Autodesk Inventor part; units mm, degrees
ref_plane "YZ Plane" through (0, 0, 0) normal (1, 0, 0) x (0, 1, 0)
ref_plane "XZ Plane" through (0, 0, 0) normal (0, 1, 0) x (-1, 0, 0)
ref_plane "XY Plane" through (0, 0, 0) normal (0, 0, 1) x (1, 0, 0)
sketch "Sketch1" plane through (0, 0, 0) normal (1, 0, 0) x (0, 1, 0)
  line L0 (0, 0) -> (0, -24)
  line L1 (0, -24) -> (20, -24)
  line L2 (20, -24) -> (20, -20.7846)
  line L3 (20, -20.7846) -> (8, 0)
  line L4 (8, 0) -> (0, 0)
  dimension "d0" = 120
  dimension "d1" = 24
  dimension "d2" = 8
  dimension "d3" = 20
extrude "Extrusion1" add sketch "Sketch1" along normal blind 32
sketch "Sketch3" plane through (0, 8, 0) normal (0, 0.866, 0.5) x (1, 0, 0)
  circle A0 centre (8, 20) radius 3.6
  circle A1 centre (24, 20) radius 3.6
  circle A2 centre (24, 4) radius 3.6
  circle A3 centre (8, 4) radius 3.6
  line L0 (0, 0) -> (32, 0)
  line L1 (32, 24) -> (32, 0)
  line L2 (0, 24) -> (32, 24)
  circle A4 centre (16, 12) radius 3.7
  point P0 (0, -4)
  dimension "d17" = 7.2
  dimension "d18" = 7.2
  dimension "d19" = 7.2
  dimension "d20" = 7.2
  dimension "d21" = 16
  dimension "d22" = 16
  dimension "d23" = 16
  dimension "d25" = 8
  dimension "d26" = 4
  dimension "d29" = 7.4
  dimension "d30" = 8
  dimension "d31" = 8
extrude "Extrusion2" cut sketch "Sketch3" against normal through all contours A0 | A1 | A2 | A3
extrude "Extrusion3" cut sketch "Sketch3" against normal blind 6 contours A4
sketch "Sketch4" plane through (0, 8, 0) normal (0, 0.866, 0.5) x (1, 0, 0)
  circle A0 centre (24, 20) radius 2
  circle A1 centre (8, 20) radius 2
  circle A2 centre (24, 4) radius 2
  circle A3 centre (8, 4) radius 2
  circle A4 centre (24, 20) radius 3.6
  circle A5 centre (8, 20) radius 3.6
  circle A6 centre (8, 4) radius 3.6
  circle A7 centre (24, 4) radius 3.6
  circle A8 centre (8, 20) radius 3.6
  circle A9 centre (24, 20) radius 3.6
  circle A10 centre (24, 4) radius 3.6
  circle A11 centre (8, 4) radius 3.6
  point P0 (0, -4)
  dimension "d34" = 4
  dimension "d35" = 4
  dimension "d36" = 4
  dimension "d37" = 4
  dimension "d38" = 7.2
  dimension "d39" = 7.2
  dimension "d40" = 7.2
  dimension "d41" = 7.2
extrude "Extrusion4" add sketch "Sketch4" against normal blind 6
sketch "Sketch7" plane through (0, 0, 0) normal (-1, 0, 0) x (0, 0, 1)
  line L0 (-24, 20) -> (-20.7846, 20)
  line L1 (-24, 20) -> (-24, 2.5)
  line L2 (-24, 0) -> (-24, 13.6308)
  line L3 (-24, 2.5) -> (0, 2.5)
  line L4 (-20.7846, 20) -> (0, 8)
  line L5 (0, 2.5) -> (0, 8)
  line L6 (0, 8) -> (-20.7846, 20)
  line L7 (-20.7846, 20) -> (-24, 20)
  point P0 (0, 0)
  dimension "d52" = 17.5
extrude "Extrusion7" add sketch "Sketch7" along normal blind 10
sketch "Sketch8" plane through (32, 0, 0) normal (1, 0, 0) x (0, 0, -1)
  line L0 (24, 20) -> (20.7846, 20)
  line L1 (24, 20) -> (24, 2.5)
  line L2 (24, 13.6308) -> (24, 0)
  line L3 (24, 2.5) -> (0, 2.5)
  line L4 (20.7846, 20) -> (0, 8)
  line L5 (0, 2.5) -> (0, 8)
  line L6 (0, 8) -> (20.7846, 20)
  line L7 (20.7846, 20) -> (24, 20)
  point P0 (0, 0)
  dimension "d55" = 17.5
extrude "Extrusion8" add sketch "Sketch8" along normal blind 10
sketch "Sketch9" plane through (0, 0, 0) normal (0, 0, 1) x (1, 0, 0)
  line L0 (-10, 8) -> (42, 8)
  line L1 (-10, 8) -> (42, 8)
  line L2 (42, 8) -> (42, -16)
  line L3 (42, -16) -> (-10, -16)
  line L4 (-10, -16) -> (-10, 8)
  point P0 (0, 0)
  dimension "d58" = 24
  dimension "d59" = 52
extrude "Extrusion9" add sketch "Sketch9" along normal blind 5
sketch "Sketch10" plane through (42, 0, 0) normal (1, 0, 0) x (0, 0, -1)
  line L0 (0, 8) -> (-8.6359, 3.0141)
  line L1 (-8.6359, 3.0141) -> (-8.6359, 11.5347)
  line L2 (-5, 8) -> (-5, -16)
  line L3 (-8.6359, 11.5347) -> (0, 11.5347)
  line L4 (0, 11.5347) -> (0, 8)
  line L5 (20.7846, 20) -> (0, 8)
  point P0 (0, 0)
  dimension "d62" = 180
extrude "Extrusion10" cut sketch "Sketch10" against normal through all
properties part number "intakemount"
Check sheet for the modelled part. Datum: model origin and axes. Units: mm. A direction names the side the tool comes from. Round coordinates to 2 decimals unless told otherwise and drop trailing zeros. Order: outer loops, then holes, each group sorted by start corner. A loop starts at its lowest first (then second) coordinate and runs counter-clockwise, first axis right, second up. Notation, with made-up numbers: M 19.25,88 L 58.25,88 A26 cw 58.25,119 Z; hole C 86.5,30 d11. An arc over 180 degrees is marked long. One line per item, written item: value. Start each with the question number.
1. Section check C-C on y = -8. Enter the section's corners in (x, z), and give its area (3 significant figures).
2. Access from +Z, -Z, +X, -X, +Y, -Y to the whole of each face (thin tool, end or side, straight path). Record for faces 1 (the flat face through (0, 1, -12)), 2 (the flat face through (37, 2.5, -12)), 3 (the flat face through (25.55, 4.03, -5.12)).
3. Release check for a two-part mould opening along X. For faces 4 (the cylindrical face through (25.908, 15.739, -19.32)), 5 (the flat face through (-5, 2.5, -12)), 6 (the flat face through (-10, 5, -10)), 7 (the cylindrical face through (9.908, 15.739, -19.32)) record: released by +X, released by -X, zero draft, split by the parting line, or undercut.
4. Scan lines: line 1 along X through (y, z) = (1, -8); line 2 along X through (y, z) = (1, -6.5); line 3 along Z through (x, y) = (37.5, -4). Record each from-to range of solid material in increasing order.
5. Section check D-D on x = 24. Enter the section's corners in (y, z), and give its area (3 significant figures).
6. Section check A-A on x = 9. Enter the section's corners in (y, z).
7. Section check B-B on x = 37.5. Enter the section's corners in (y, z).
8. Gauge pin test, flat ends, axial feed: P1, Ø3, axis at x = -2.5, z = -6.5, coming from the -Y side; P2, Ø0.8, axis at y = 1.5, z = -6, coming from the -X side; P3, Ø10, axis at x = 30.5, z = -8.5, coming from the -Y side; P4, Ø20.5, axis at x = 9, y = -3.5, coming from the -Z side. Record the tip position at first contact, or that the pin passes through.
Results found:
1. outline: M -10,0 L 42,0 L 42,5 L -10,5 Z
1. area: 260 mm^2
2. face 1: -Z, -X, -Y
2. face 2: -Z, +X, -Y
2. face 3: none
3. face 4: undercut
3. face 5: zero draft
3. face 6: released by -X
3. face 7: undercut
4. line 1: 0 to 4.45, 11.55 to 20.45, 27.55 to 32
4. line 2: 0 to 4.92, 11.08 to 20.92, 27.08 to 32
4. line 3: 0 to 5
5. outline: M -16,0 L 0,0 L 0,-5.08 L 3,-3.35 L 3.8,-4.73 L 9,-1.73 L 8.2,-0.35 L 8,0 L 5.11,5 L -16,5 Z; M 0,-23.56 L 11,-17.2 L 11.8,-18.59 L 17,-15.59 L 16.2,-14.2 L 11.8,-6.58 L 11,-5.2 L 5.8,-8.2 L 6.6,-9.58 L 0,-13.39 Z; M 13.63,-24 L 20,-24 L 20,-20.78 L 19.8,-20.44 L 19,-19.05 L 13.8,-22.05 L 14.6,-23.44 Z
5. area: 327 mm^2
6. outline: M -16,0 L 0,0 L 0,-5.24 L 3.07,-3.47 L 3.94,-4.96 L 9.13,-1.96 L 8.27,-0.47 L 8,0 L 5.11,5 L -16,5 Z; M 0,-23.72 L 11.07,-17.33 L 11.94,-18.82 L 17.13,-15.82 L 16.27,-14.33 L 11.73,-6.46 L 10.87,-4.96 L 5.67,-7.96 L 6.53,-9.46 L 0,-13.23 Z; M 13.35,-24 L 20,-24 L 20,-20.78 L 19.73,-20.32 L 18.87,-18.82 L 13.67,-21.82 L 14.53,-23.32 Z
7. outline: M -16,0 L 2.5,0 L 2.5,-24 L 20,-24 L 20,-20.78 L 8,0 L 5.11,5 L -16,5 Z
8. P1: y = 2.5
8. P2: x = 0
8. P3: y = 0
8. P4: z = -24
